from build123d import *

# Parameters (mm, degrees)
SKETCH1_W           = 9
SKETCH1_H           = 9
BOSS_EXTRUDE1_DEPTH = 116.15
SKETCH2_W           = 3.175
SKETCH2_H           = 117
BOSS_EXTRUDE2_DEPTH = 4.5


with BuildPart() as part:
    # Sketch1 → Boss-Extrude1 (new body, symmetric)
    with BuildSketch(Plane.XY):
        Rectangle(SKETCH1_W, SKETCH1_H)
    extrude(amount=BOSS_EXTRUDE1_DEPTH, both=True)

    # Sketch2 → Boss-Extrude2 (add, symmetric)
    with BuildSketch(Plane(origin=(0, 0, 0), x_dir=(1, 0, 0), z_dir=(0, 1, 0))):
        with Locations((6.0875, 0)):
            Rectangle(SKETCH2_W, SKETCH2_H)
        with Locations((-6.0875, 0)):
            Rectangle(SKETCH2_W, SKETCH2_H)
    extrude(amount=BOSS_EXTRUDE2_DEPTH, both=True)


solid = part.part
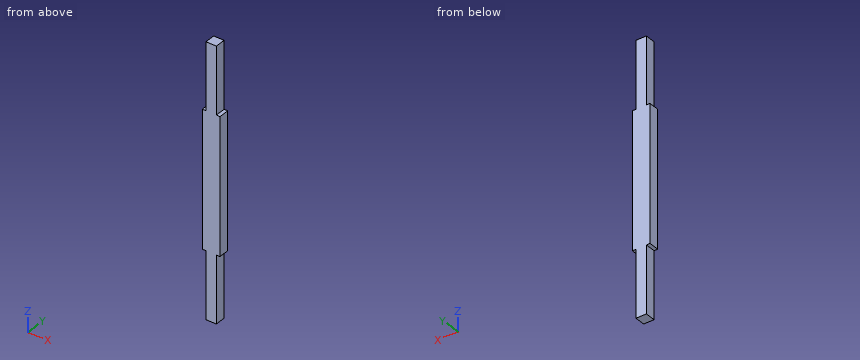
Design review of the part built by this model. Coordinates are the model's own, in mm. Coordinates: 2 decimals unless noted, no trailing zeros. Loops run counter-clockwise (first coordinate to the right, second up) from the corner with the lowest first, then second, coordinate; pieces in that order, holes last. Notation, with made-up numbers: (14, 69) -> (59, 69) arc R24 ccw to (59, 79) -> close; hole circle Ø4 at (48.25, 0.25). An arc over 180 degrees is marked (long way). Use a Markdown table: item, result. Add a question column.
Item 1: Wall thickness on L1, parallel to Z at x = -5.25, y = -3.25; L2, parallel to X at y = -0.75, z = -105: over which ranges is each line inside the solid? List them lowest first. Write a range as from..to.
Item 2: We need section B-B, the plane z = 99. Write out the cut boundary in (x, y).
Item 3: Clearance check with flat-ended pins moving along their axes: P1, Ø1.5, axis at y = -3.5, z = -69.5, coming from the -X side; P2, Ø1.6, axis at x = 5.5, y = 2, coming from the +Z side; P3, Ø1.6, axis at x = 5.5, y = -1.5, coming from the -Z side. State where each tip first meets the part, or that it passes through.
Item 4: We need section A-A, the plane y = 2. Write out the cut boundary in (x, z) (3 decimals).
Numbers:
| question | item | result |
|---|---|---|
| 1 | L1 | z = -58.5..58.5 |
| 1 | L2 | x = -4.5..4.5 |
| 2 | outline | (-4.5, -4.5) -> (4.5, -4.5) -> (4.5, 4.5) -> (-4.5, 4.5) -> close |
| 3 | P1 | stops at x = -4.5 |
| 3 | P2 | stops at z = 58.5 |
| 3 | P3 | stops at z = -58.5 |
| 4 | outline | (-7.675, -58.5) -> (-4.5, -58.5) -> (-4.5, -116.15) -> (4.5, -116.15) -> (4.5, -58.5) -> (7.675, -58.5) -> (7.675, 58.5) -> (4.5, 58.5) -> (4.5, 116.15) -> (-4.5, 116.15) -> (-4.5, 58.5) -> (-7.675, 58.5) -> close |
